Input: part model. Units: mm. Frame: model coordinates. Coordinates: 2 decimals unless noted, no trailing zeros. Loops run counter-clockwise (first coordinate to the right, second up) from the corner with the lowest first, then second, coordinate; pieces in that order, holes last.
```python
from build123d import *

# Parameters (mm, degrees)
F0_W     = 3.556
F0_H     = 1.5875
F1_DEPTH = 3.175


with BuildPart() as f1:
    # F0 (on Top) → F1 (new body)
    with BuildSketch(Plane.XY):
        with Locations((-43.68662, 21.858571)):
            Rectangle(F0_W, F0_H)
        with Locations((-43.68662, 14.556071)):
            Rectangle(F0_W, F0_H)
        Polygon((43.43538, 23.922321), (-41.90862, 23.922321), (-41.90862, 22.652321), (-41.90862, 21.064821), (-41.90862, 19.858321), (-35.81262, 19.858321), (-35.81262, 22.398321), (-33.01862, 22.398321), (-33.01862, 19.858321), (-31.836697, 19.858321), (-31.836697, 18.207321), (-31.836697, 16.556321), (-33.01862, 16.556321), (-33.01862, 14.016321), (-35.81262, 14.016321), (-35.81262, 16.556321), (-41.90862, 16.556321), (-41.90862, 15.349821), (-41.90862, 13.762321), (-41.90862, 12.492321), (43.43538, 12.492321), align=None)
    extrude(amount=F1_DEPTH)


solid = f1.part
```
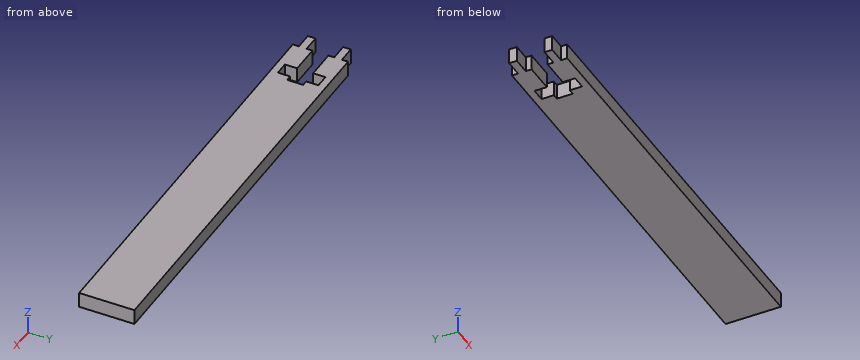
Item 1: Section query A-A (z = 0.6). Output: boundary loops of the cut face in (x, y), then the cut area to 3 significant figures.
Result:
outline: (-45.46, 13.76) - (-41.91, 13.76) - (-41.91, 12.49) - (43.44, 12.49) - (43.44, 23.92) - (-41.91, 23.92) - (-41.91, 22.65) - (-45.46, 22.65) - (-45.46, 21.06) - (-41.91, 21.06) - (-41.91, 19.86) - (-35.81, 19.86) - (-35.81, 22.4) - (-33.02, 22.4) - (-33.02, 19.86) - (-31.84, 19.86) - (-31.84, 16.56) - (-33.02, 16.56) - (-33.02, 14.02) - (-35.81, 14.02) - (-35.81, 16.56) - (-41.91, 16.56) - (-41.91, 15.35) - (-45.46, 15.35) - close
area: 939 mm2
Item 2: Line query: L1, parallel to X at y = 15, z = 3; L2, parallel to Y at x = -32, z = 2.5; L3, parallel to X at y = 19.75, z = 0.7. Output: solid intervals per line, ascending.
Result:
L1: x = -45.46 to -35.81, -33.02 to 43.44
L2: y = 12.49 to 16.56, 19.86 to 23.92
L3: x = -31.84 to 43.44
Item 3: Section query B-B (y = 19). Output: boundary loops of the cut face in (x, z) (3 decimals), then the cut area to 3 significant figures.
Result:
outline: (-31.837, 0) - (43.435, 0) - (43.435, 3.175) - (-31.837, 3.175) - close
area: 239 mm2
Item 4: Contact query for flat-ended pins moving along their axis: P1, Ø1.6, axis at y = 18.5, z = 1.5, coming from the -X side; P2, Ø0.6, axis at y = 13, z = 2, coming from the -X side. Output: stop coordinate, or through.
Result:
P1: stops at x = -31.84
P2: stops at x = -41.91
